```python
from build123d import *

# Parameters (mm, degrees)
SKETCH_1_W          = 6
SKETCH_1_H          = 8
SKETCH_1_R          = 2
EXTRUDE_1_DEPTH     = 2
SKETCH_2_W          = 6
SKETCH_2_H          = 12
SKETCH_2_R          = 1.65
EXTRUDE_2_DEPTH     = 2
SKETCH_3_W          = 10
SKETCH_3_H          = 2
EXTRUDE_3_DEPTH     = 6
SKETCH_4_W          = 10
SKETCH_4_H          = 2
EXTRUDE_4_DEPTH     = 6
SKETCH_6_R          = 1.65
CUT_EXTRUDE_1_DEPTH = 6


with BuildPart() as part:
    # 草图1 → 凸台-拉伸1 (new body)
    with BuildSketch(Plane.XY):
        with Locations((0, 1)):
            Rectangle(SKETCH_1_W, SKETCH_1_H)
        Circle(SKETCH_1_R, mode=Mode.SUBTRACT)
    extrude(amount=EXTRUDE_1_DEPTH)

    # 草图2 → 凸台-拉伸2 (add)
    with BuildSketch(Plane(origin=(0, 5, 0), x_dir=(1, 0, 0), z_dir=(0, 1, 0))):
        with Locations((0, 4)):
            Rectangle(SKETCH_2_W, SKETCH_2_H)
        with Locations(Location((0, 7, 0), (0, 0, 270))):
            Circle(SKETCH_2_R, mode=Mode.SUBTRACT)
    extrude(amount=EXTRUDE_2_DEPTH)

    # 草图3 → 凸台-拉伸3 (add)
    with BuildSketch(Plane.ZY.offset(3)):
        with Locations((-5, 6)):
            Rectangle(SKETCH_3_W, SKETCH_3_H)
    extrude(amount=EXTRUDE_3_DEPTH)

    # 草图4 → 凸台-拉伸4 (add)
    with BuildSketch(Plane(origin=(3, 0, 0), x_dir=(0, 0, -1), z_dir=(1, 0, 0))):
        with Locations((5, 6)):
            Rectangle(SKETCH_4_W, SKETCH_4_H)
    extrude(amount=EXTRUDE_4_DEPTH)

    # 草图6 → 切除-拉伸1 (cut)
    with BuildSketch(Plane(origin=(0, 7, 0), x_dir=(1, 0, 0), z_dir=(0, 1, 0))):
        with Locations(Location((-6.5, 7, 0), (0, 0, 270))):
            Circle(SKETCH_6_R)
        with Locations(Location((6.5, 7, 0), (0, 0, 270))):
            Circle(SKETCH_6_R)
    extrude(amount=-CUT_EXTRUDE_1_DEPTH, mode=Mode.SUBTRACT)


solid = part.part
```
Verification items for the finished model (mm, model axes). A direction names the side the tool comes from. Give positions to 0.01 mm unless a question says otherwise; leave off trailing zeros. Order: outer loops, then holes, each group sorted by start corner. A loop starts at its lowest first (then second) coordinate and runs counter-clockwise, first axis right, second up. Notation, with made-up numbers: M 77,-29.5 L 100,-29.5 A27 cw 100,-11.5 Z; hole C -35,6.25 d6. An arc over 180 degrees is marked long. Return JSON: item names as keys, results as strings. Group by question number.
1) Mould release check, pull along X, two halves, no side actions. Record for faces 4 (the face through (0, -3, 1)), 5 (the face through (-3, 2, 1)), 6 (the face through (9, 6, -5)), 7 (the face through (0.07, 5.99, -8.65)): pulls with the +X half, pulls with the -X half, needs draft (parallel to the pull), parting line crosses it, or undercut.
2) Scan lines: line 1 (X direction, y = 6.5, z = -7); line 2 (Y direction, x = 8.25, z = -4.5); line 3 (Y direction, x = 0, z = 0.5). Record each from-to range of solid material in increasing order.
3) Section check B-B on x = -6.5. Record the cut outline in (y, z), and give its area (3 significant figures).
4) Section check D-D on y = 2.5. Record the cut outline in (x, z), and give its area (3 significant figures).
5) Section check A-A on z = -7. Record the cut outline in (x, y), and give its area (3 significant figures).
6) Section check C-C on y = -1. Record the cut outline in (x, z).
7) Go/stop test with flat-tipped pins: pin 1 Ø1.6 at (y, z) = (3.5, 1.5) entering from +X; pin 2 Ø1.8 at (x, y) = (1, 1.5) entering from -Z; pin 3 Ø4 at (x, z) = (6.5, -7) entering from +Y; pin 4 Ø1 at (y, z) = (3.5, 1) entering from -X. Record where each tip stops, or that it passes through.
8) Access from +Z, -Z, +X, -X, +Y, -Y to the whole of each face (thin tool, end or side, straight path). Record for faces 1 (the face through (0, 5, -5)), 2 (the face through (-6, 6, 0)), 3 (the face through (6, 6, 0)).
Answer block:
{
 "1": {"face 4": "needs draft", "face 5": "pulls with the -X half", "face 6": "pulls with the +X half", "face 7": "undercut"},
 "2": {"line 1": "x = -9 to -8.15, -4.85 to -1.65, 1.65 to 4.85, 8.15 to 9", "line 2": "y = 5 to 7", "line 3": "y = -3 to -2, 2 to 7"},
 "3": {"outline": "M 5,-10 L 7,-10 L 7,-8.65 L 5,-8.65 Z; M 5,-5.35 L 7,-5.35 L 7,0 L 5,0 Z", "area": "13.4 mm^2"},
 "4": {"outline": "M -3,0 L 3,0 L 3,2 L -3,2 Z", "area": "12.0 mm^2"},
 "5": {"outline": "M -9,5 L -8.15,5 L -8.15,7 L -9,7 Z; M -4.85,5 L -1.65,5 L -1.65,7 L -4.85,7 Z; M 1.65,5 L 4.85,5 L 4.85,7 L 1.65,7 Z; M 8.15,5 L 9,5 L 9,7 L 8.15,7 Z", "area": "16.2 mm^2"},
 "6": {"outline": "M -3,0 L -1.73,0 L -1.73,2 L -3,2 Z; M 1.73,0 L 3,0 L 3,2 L 1.73,2 Z"},
 "7": {"pin 1": "stops at x = 3", "pin 2": "stops at z = 0", "pin 3": "stops at y = 7", "pin 4": "stops at x = -3"},
 "8": {"face 1": "-Z, +X, -X, -Y", "face 2": "+Z, -X, +Y, -Y", "face 3": "+Z, +X, +Y, -Y"}
}
